For this review, take the finished solid that the model builds, in its own axes (mm). Face numbers are marked on the shaded views. A direction names the side the tool comes from. Round coordinates to 2 decimals unless told otherwise and drop trailing zeros. Order: outer loops, then holes, each group sorted by start corner. A loop starts at its lowest first (then second) coordinate and runs counter-clockwise, first axis right, second up.
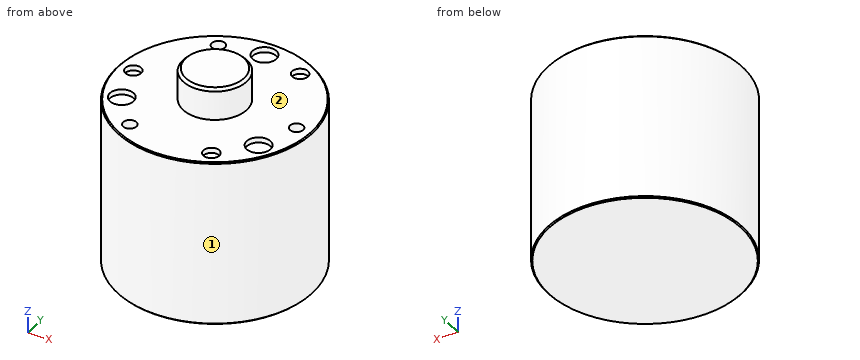
```python
from build123d import *

# Parameters (mm, degrees)
F0_R      = 18.35
F1_DEPTH  = 31.4
F2_R      = 6
F3_DEPTH  = 6
F4_SIZE   = 0.5
F5_SIZE   = 0.2
F6_R      = 2.25
F7_DEPTH  = 1
F9_D      = 3
F9_DEPTH  = 1
F9_TIP    = 0.9012909285
F11_D     = 2.5
F11_DEPTH = 3.8
F11_TIP   = 0.7510757738


with BuildPart() as f1:
    # F0 (on Top) → F1 (new body)
    with BuildSketch(Plane.XY):
        Circle(F0_R)
    extrude(amount=-F1_DEPTH)

    # F2 (on Top) → F3 (join)
    with BuildSketch(Plane.XY):
        Circle(F2_R)
    extrude(amount=F3_DEPTH)

    # F4
    f4_edges = [f1.edges().sort_by_distance(p)[0] for p in [
        (-6, 0, 6),
    ]]
    chamfer(f4_edges, length=F4_SIZE)

    # F5
    f5_edges = [f1.edges().sort_by_distance(p)[0] for p in [
        (-18.35, 0, 0),
        (-18.35, 0, -31.4),
    ]]
    chamfer(f5_edges, length=F5_SIZE)

    # F6 (on Top) → F7 (cut)
    with BuildSketch(Plane.XY):
        with Locations((0, 15)):
            Circle(F6_R)
        with Locations((-12.9903810568, -7.5)):
            Circle(F6_R)
        with Locations((12.9903810568, -7.5)):
            Circle(F6_R)
    extrude(amount=-F7_DEPTH, mode=Mode.SUBTRACT)

    # F9
    with Locations(Plane.XY):
        with Locations((7.75, 13.4233937587), (7.75, -13.4233937587), (-15.5, 0)):
            Hole(F9_D / 2, depth=F9_DEPTH)
            with Locations((0, 0, -(F9_DEPTH + F9_TIP / 2))):  # 118° drill point
                Cone(0, F9_D / 2, F9_TIP, mode=Mode.SUBTRACT)

    # F11
    with Locations(Plane.XY):
        with Locations((-7.75, 13.4233937587), (15.5, 0), (-7.75, -13.4233937587)):
            Hole(F11_D / 2, depth=F11_DEPTH)
            with Locations((0, 0, -(F11_DEPTH + F11_TIP / 2))):  # 118° drill point
                Cone(0, F11_D / 2, F11_TIP, mode=Mode.SUBTRACT)


solid = f1.part
```
Q1. Tool access review of the marked faces 1 and 2: name each direction out of +Z, -Z, +X, -X, +Y, -Y from which nothing blocks a thin tool from reaching the whole face with its end or side.
Q2. Clearance check with flat-ended pins moving along their axes: pin 1 (3.5 mm diameter, centred on x = 7.75, y = -13.42, fed in from +Z); pin 2 (3 mm diameter, centred on x = -6.5, z = -20, fed in from +Y); pin 3 (2 mm diameter, centred on x = 0, y = 15, fed in from +Z). State where each tip first meets the part, or that it passes through.
Q3. Wall thickness on line 1 (Y direction, x = -7, z = -1); line 2 (Z direction, x = -15.5, y = -8); line 3 (Y direction, x = 7.75, z = -0.45): over which ranges is each line inside the solid? List them lowest first.
Q4. Take a section at A-A, the plane z = -20.5. State the section outline as (x, y) points, plus the area to 3 significant figures.
Working result:
1. face 1: +Z, -Z
1. face 2: +Z
2. pin 1: stops at z = 0
2. pin 2: stops at y = 17.66
2. pin 3: stops at z = -1
3. line 1: y = -16.96 to -14.42, -12.42 to 12.42, 14.42 to 16.96
3. line 2: z = -31.4 to 0
3. line 3: y = -16.63 to -14.92, -11.92 to 11.92, 14.92 to 16.63
4. outline: circle Ø36.7 at (0, 0)
4. area: 1,060 mm2
